from build123d import *

# Parameters (mm, degrees)
SKETCH1_R           = 8
BOSS_EXTRUDE1_DEPTH = 7.5
BOSS_EXTRUDE2_DEPTH = 7.7
SKETCH3_R           = 8
BOSS_EXTRUDE3_DEPTH = 1.5
SKETCH4_R           = 4
CUT_EXTRUDE2_DEPTH  = 17.5


with BuildPart() as part:
    # Sketch1 → Boss-Extrude1 (new body)
    with BuildSketch(Plane.XY):
        Circle(SKETCH1_R)
    extrude(amount=BOSS_EXTRUDE1_DEPTH)

    # Sketch2 → Boss-Extrude2 (add)
    with BuildSketch(Plane.XY.offset(7.5)):
        Polygon((-0.820372416, 5.179627584), (0, 6), (0.820372416, 5.179627584), (1.854101966, 5.706339098), (2.38081348, 4.672609548), (3.526711514, 4.854101966), (3.708203932, 3.708203933), (4.854101966, 3.526711514), (4.672609548, 2.38081348), (5.706339098, 1.854101966), (5.179627584, 0.820372416), (6, 0), (5.179627584, -0.820372416), (5.706339098, -1.854101966), (4.672609548, -2.38081348), (4.854101966, -3.526711514), (3.708203933, -3.708203932), (3.526711514, -4.854101966), (2.38081348, -4.672609548), (1.854101966, -5.706339098), (0.820372416, -5.179627584), (0, -6), (-0.820372416, -5.179627584), (-1.854101966, -5.706339098), (-2.38081348, -4.672609548), (-3.526711514, -4.854101966), (-3.708203932, -3.708203932), (-4.854101966, -3.526711514), (-4.672609548, -2.38081348), (-5.706339098, -1.854101966), (-5.179627584, -0.820372416), (-6, 0), (-5.179627584, 0.820372416), (-5.706339098, 1.854101966), (-4.672609548, 2.38081348), (-4.854101966, 3.526711514), (-3.708203932, 3.708203932), (-3.526711514, 4.854101966), (-2.38081348, 4.672609548), (-1.854101966, 5.706339098), align=None)
    extrude(amount=BOSS_EXTRUDE2_DEPTH)

    # Sketch3 → Boss-Extrude3 (add)
    with BuildSketch(Plane.XY.offset(15.2)):
        Circle(SKETCH3_R)
    extrude(amount=BOSS_EXTRUDE3_DEPTH)

    # Sketch4 → Cut-Extrude2 (cut)
    with BuildSketch(Plane.XY.offset(16.7)):
        Circle(SKETCH4_R)
    extrude(amount=-CUT_EXTRUDE2_DEPTH, mode=Mode.SUBTRACT)


solid = part.part
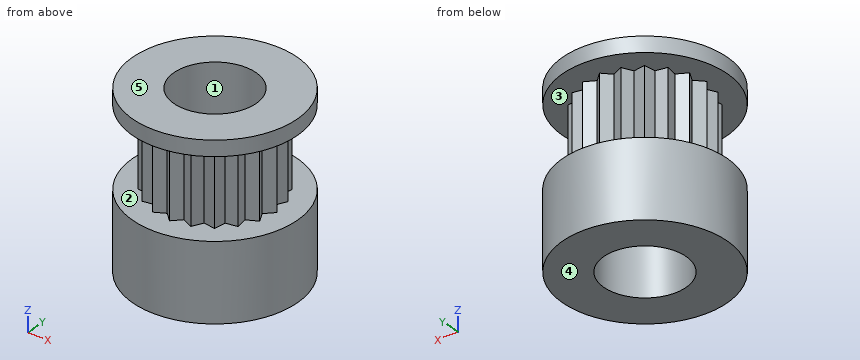
CAD build for the part. Positions are in the model's coordinates, mm. Face numbers are marked on the shaded views. A direction names the side the tool comes from. Round coordinates to 2 decimals unless told otherwise and drop trailing zeros. Put each result on its own line as item: value. Start each with the question number.
1) Drill centre lines: probe 1 along Z at (x, y) = (5, 3.5); probe 2 along Y at (x, z) = (0, 5); probe 3 along Y at (x, z) = (3.25, 14). Where is each one in solid material? Low to high. Write a range as [from, to].
2) 3-axis set-ups, long thin cutter, end or side, ignore diameter. For the marked faces 1 and 2: which of +Z, -Z, +X, -X, +Y, -Y reach the whole face in a straight line?
3) Pin check, flat tips, straight feed: pin 1 Ø1 at (y, z) = (-5, 15) entering from +X; pin 2 Ø1.5 at (x, z) = (-6, 7) entering from -Y; pin 3 Ø1.5 at (x, z) = (5.5, 9) entering from +Y. Stop position of each tip, or through.
4) Pull direction Z, two halves, no side cores. Call the marked faces 3, 4 and 5: pulls with the +Z half, pulls with the -Z half, needs draft (parallel to the pull), parting line crosses it, or undercut.
Resolved:
1. probe 1: [0, 7.5], [15.2, 16.7]
1. probe 2: [-8, -4], [4, 8]
1. probe 3: [-4.81, -2.33], [2.33, 4.81]
2. face 1: +Z, -Z
2. face 2: none
3. pin 1: x = 6.59
3. pin 2: y = -6.04
3. pin 3: y = 3.54
4. face 3: undercut
4. face 4: pulls with the -Z half
4. face 5: pulls with the +Z half
